Can you work these out from the model? Positions are in its coordinate system, mm. Coordinates: 2 decimals unless noted, no trailing zeros. Loops run counter-clockwise (first coordinate to the right, second up) from the corner with the lowest first, then second, coordinate; pieces in that order, holes last.
```python
from build123d import *

# Parameters (mm, degrees)
F1_DEPTH = 1
F2_R     = 10
F4_D     = 9
F5_D     = 6.6


with BuildPart() as f1:
    # F0 (on Top) → F1 (new body)
    with BuildSketch(Plane.XY):
        with BuildLine():
            Line((10.468547, 0), (5.79805, 17.543572))
            ThreePointArc((5.79805, 17.543572), (0, 22), (-5.79805, 17.543572))
            Line((-5.79805, 17.543572), (-10.468547, 0))
            Line((-10.468547, 0), (-5.79805, -17.543572))
            ThreePointArc((-5.79805, -17.543572), (0, -22), (5.79805, -17.543572))
            Line((5.79805, -17.543572), (10.468547, 0))
        make_face()
    extrude(amount=F1_DEPTH)

    # F2
    f2_edges = [f1.edges().sort_by_distance(p)[0] for p in [
        (10.468547, 0, 0.5),
        (-10.468547, 0, 0.5),
    ]]
    fillet(f2_edges, radius=F2_R)

    # F4 (through all)
    with Locations(Plane.XY.offset(1)):
        with Locations((0, 0)):
            Hole(F4_D / 2)

    # F5 (through all)
    with Locations(Plane.XY.offset(1)):
        with Locations((0, 16), (0, -16)):
            Hole(F5_D / 2)


solid = f1.part
```
Item 1: We'd pull the mould along Y, two halves only. Please class faces 1 (the face through (2.43, 18.23, 0.49)), 2 (the face through (0, -5, 0)), 3 (the face through (10.12, 0.04, 0.51)): +Y half, -Y half, draft (parallel to the pull), parting line (faces both ways), or undercut.
Results are:
face 1: undercut
face 2: draft
face 3: parting line
Item 2: I need wall thicknesses on line 1 along Y through (x, z) = (2.75, 0.2); line 2 along X through (y, z) = (17, 0.1); line 3 along X through (y, z) = (-16.5, 0.8). Which ranges of each line are inside material? Lowest first, please.
Results are:
line 1: y = -21.33 to -17.82, -14.18 to -3.56, 3.56 to 14.18, 17.82 to 21.33
line 2: x = -5.94 to -3.14, 3.14 to 5.94
line 3: x = -6.08 to -3.26, 3.26 to 6.08
Item 3: Suppose I cut it at D-D, the plane x = -2.75. Please give me the cut outline in (y, z), plus the area to 3 significant figures.
Results are:
outline: (-21.33, 0) - (-17.82, 0) - (-17.82, 1) - (-21.33, 1) - close; (-14.18, 0) - (-3.56, 0) - (-3.56, 1) - (-14.18, 1) - close; (3.56, 0) - (14.18, 0) - (14.18, 1) - (3.56, 1) - close; (17.82, 0) - (21.33, 0) - (21.33, 1) - (17.82, 1) - close
area: 28.2 mm2
Item 4: Suppose I cut it at A-A, the plane y = 0. Please give me the cut outline in (x, z), plus the area to 3 significant figures.
Results are:
outline: (-10.12, 0) - (-4.5, 0) - (-4.5, 1) - (-10.12, 1) - close; (4.5, 0) - (10.12, 0) - (10.12, 1) - (4.5, 1) - close
area: 11.2 mm2
Item 5: Suppose I cut it at B-B, the plane z = 0.4. Please give me the cut outline in (x, y).
Results are:
outline: (-9.78, -2.57) - (-5.8, -17.54) arc R6 ccw to (5.8, -17.54) - (9.78, -2.57) arc R10 ccw to (9.78, 2.57) - (5.8, 17.54) arc R6 ccw to (-5.8, 17.54) - (-9.78, 2.57) arc R10 ccw to start; hole circle Ø9 at (0, 0); hole circle Ø6.6 at (0, -16); hole circle Ø6.6 at (0, 16)
Item 6: Suppose I cut it at C-C, the plane x = 0. Please give me the cut outline in (y, z).
Results are:
outline: (-22, 0) - (-19.3, 0) - (-19.3, 1) - (-22, 1) - close; (-12.7, 0) - (-4.5, 0) - (-4.5, 1) - (-12.7, 1) - close; (4.5, 0) - (12.7, 0) - (12.7, 1) - (4.5, 1) - close; (19.3, 0) - (22, 0) - (22, 1) - (19.3, 1) - close
